Geometry check sheet. Reference: the model listing, model coordinates, mm. Face numbers are marked on the shaded views. A direction names the side the tool comes from. Give positions to 0.01 mm unless a question says otherwise; leave off trailing zeros. Order: outer loops, then holes, each group sorted by start corner. A loop starts at its lowest first (then second) coordinate and runs counter-clockwise, first axis right, second up. Notation, with made-up numbers: M 35,-1 L 68,-1 A23 cw 68,19 Z; hole C -29.75,38.25 d10. An arc over 180 degrees is marked long. Put each result on its own line as item: value. Start each with the question number.
Q1. Section check B-B on z = -8. Record the cut outline in (x, y), then the cut area to 3 significant figures.
Q2. Material ranges on L1, parallel to X at y = 87, z = -15.5; L2, parallel to X at y = 87, z = -22; L3, parallel to Y at x = 1, z = 1, recorded low to high.
Q3. Go/stop test with flat-tipped pins: pin 1 (6 mm diameter, centred on y = 72.5, z = 5.5, fed in from -X); pin 2 (12 mm diameter, centred on x = 27.5, z = -18.5, fed in from +Y); pin 3 (1 mm diameter, centred on x = 40, y = 56.5, fed in from -Z). Record where each tip stops, or that it passes through.
Q4. Mould release check, pull along X, two halves, no side actions. Record for the marked faces 4, 5, 6 and 7: +X half, -X half, draft (parallel to the pull), parting line (faces both ways), or undercut.
Q5. Access from +Z, -Z, +X, -X, +Y, -Y to the whole of each face (thin tool, end or side, straight path). Record for the marked faces 1, 2 and 3.
Q6. Section check C-C on x = -34.5. Record the cut outline in (y, z), then the cut area to 3 significant figures.
Q7. Section check A-A on y = 38. Record the cut outline in (x, z).
Q8. Section check D-D on x = -14.5. Record the cut outline in (y, z).
```python
from build123d import *

# Parameters (mm, degrees)
EXTRUDE_2_DEPTH          = 90
CUT_EXTRUDE_1_DEPTH      = 114.317207464
CUT_EXTRUDE_1_DEPTH_BACK = 114.317207464
EXTRUDE_3_DEPTH          = 8
SKETCH_8_OUTSIDE_W       = 163.572
SKETCH_8_OUTSIDE_H       = 147.98
SKETCH_8_OUTSIDE_W_2     = 117.820012314
SKETCH_8_OUTSIDE_H_2     = 106.962978805
CUT_EXTRUDE_2_DEPTH      = 117.531399887
SKETCH_9_R               = 2
CUT_EXTRUDE_3_DEPTH      = 115.369004136
SKETCH_10_W              = 117.820012314
SKETCH_10_H              = 8
CUT_EXTRUDE_4_DEPTH      = 20
CUT_EXTRUDE_6_DEPTH      = 5
CHAMFER_1_SIZE           = 8


with BuildPart() as part:
    # 草图5 → 拉伸-薄壁2 (new body)
    with BuildSketch(Plane(origin=(0, 0, 0), x_dir=(1, 0, 0), z_dir=(0, 1, 0))):
        Polygon((-58.910006157, 27.470187013), (0, 0), (58.910006157, 27.470187013), (63.136188775, 18.407109143), (0, -11.03377919), (-63.136188775, 18.407109143), align=None)
    extrude(amount=EXTRUDE_2_DEPTH)

    # 草图6 → 切除-拉伸1 (cut, two sides: drawn at the far end of the back side and taken through both)
    with BuildSketch(Plane(origin=(0, 0, 0), x_dir=(0, 0, -1), z_dir=(1, 0, 0)).offset(-CUT_EXTRUDE_1_DEPTH_BACK)):
        Polygon((-11.03377919, 0), (27.470187013, 26.960767386), (27.470187013, 0), align=None)
        Polygon((27.470187013, 90), (-11.03377919, 63.039232614), (-11.03377919, 90), align=None)
    extrude(amount=CUT_EXTRUDE_1_DEPTH + CUT_EXTRUDE_1_DEPTH_BACK, mode=Mode.SUBTRACT)

    # 草图7 → 凸台-拉伸3 (add)
    with BuildSketch(Plane(origin=(0, 47.484140436, 33.248753079), x_dir=(1, 0, 0), z_dir=(0, 0.8191520442889949, 0.5735764363510419))):
        Polygon((63.136188775, 63.06016396), (58.910006157, 74.12413912), (58.910006157, 94.12413912), (-58.910006157, 94.12413912), (-58.910006157, 74.12413912), (-63.136188775, 63.06016396), (0, 27.119475614), align=None)
    extrude(amount=EXTRUDE_3_DEPTH)

    # 草图8 outside → 切除-拉伸2 (cut, through all)
    with BuildSketch(Plane(origin=(0, 54.03735679, 37.837364569), x_dir=(1, 0, 0), z_dir=(0, 0.8191520442889948, 0.5735764363510418))):
        with Locations((0, 42.543)):
            Rectangle(SKETCH_8_OUTSIDE_W, SKETCH_8_OUTSIDE_H)
        with Locations((0, 40.642649718)):
            Rectangle(SKETCH_8_OUTSIDE_W_2, SKETCH_8_OUTSIDE_H_2, mode=Mode.SUBTRACT)
    extrude(amount=-CUT_EXTRUDE_2_DEPTH, mode=Mode.SUBTRACT)

    # 草图9 → 切除-拉伸3 (cut, through all)
    with BuildSketch(Plane(origin=(0, 47.484140436, 33.248753079), x_dir=(1, 0, 0), z_dir=(0, -0.8191520442889949, -0.5735764363510419))):
        with Locations(Location((-45, -74.12413912, 0), (0, 0, 270))):
            Circle(SKETCH_9_R)
        with Locations(Location((45, -74.12413912, 0), (0, 0, 270))):
            Circle(SKETCH_9_R)
    extrude(amount=-CUT_EXTRUDE_3_DEPTH, mode=Mode.SUBTRACT)

    # 草图10 → 切除-拉伸4 (cut)
    with BuildSketch(Plane(origin=(0, 47.484140436, 33.248753079), x_dir=(1, 0, 0), z_dir=(0, -0.8191520442889949, -0.5735764363510419))):
        with Locations((0, -90.12413912)):
            Rectangle(SKETCH_10_W, SKETCH_10_H)
    extrude(amount=-CUT_EXTRUDE_4_DEPTH, mode=Mode.SUBTRACT)

    # 草图11 → 切除-拉伸6 (cut)
    with BuildSketch(Plane(origin=(0, 47.484140436, 33.248753079), x_dir=(1, 0, 0), z_dir=(0, -0.8191520442889949, -0.5735764363510419))):
        Polygon((-58.910006157, -86.12413912), (58.910006157, -86.12413912), (58.910006157, -74.12413912), (0, -40.589232866), (-58.910006157, -74.12413912), align=None)
    extrude(amount=-CUT_EXTRUDE_6_DEPTH, mode=Mode.SUBTRACT)

    # 倒角1
    chamfer_1_edges = [part.edges().sort_by_distance(p)[0] for p in [
        (-58.910006157, 102.207405524, -33.571764708),
        (58.910006157, 102.207405524, -33.571764708),
    ]]
    chamfer(chamfer_1_edges, length=CHAMFER_1_SIZE)


solid = part.part
```
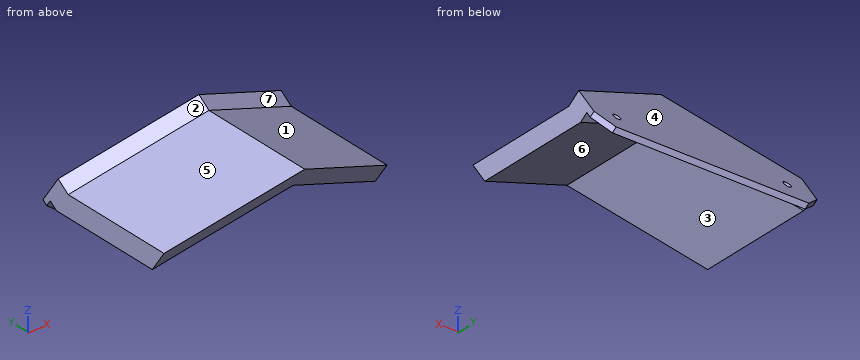
Results found:
1. outline: M -50.66,86.13 L -40.82,76.37 L -40.82,13.33 L -17.16,13.33 L -17.16,76.37 L -23.31,82.47 L 23.31,82.47 L 17.16,76.37 L 17.16,13.33 L 40.82,13.33 L 40.82,76.37 L 50.66,86.13 Z
1. area: 3,630 mm^2
2. L1: x = -58.91 to -38.66, 38.66 to 58.91
2. L2: x = -58.91 to -48.02, 48.02 to 58.91
2. L3: y = 7.03 to 73.19, 76.17 to 79.83
3. pin 1: stops at x = -22.77
3. pin 2: stops at y = 97.69
3. pin 3: stops at z = -18.89
4. face 4: draft
4. face 5: -X half
4. face 6: undercut
4. face 7: +X half
5. face 1: +Z, +X, -Y
5. face 2: +Z, -X, -Y
5. face 3: -Z, -Y
6. outline: M 11.26,-5.05 L 18.99,-16.09 L 82.03,-16.09 L 86.13,-13.22 L 100.98,-34.43 L 103.44,-32.71 L 80.86,-0.47 L 74.3,-5.05 Z
6. area: 881 mm^2
7. outline: M -58.91,-27.47 L 0,0 L 58.91,-27.47 L 58.91,-16.44 L 0,11.03 L -58.91,-16.44 Z
8. outline: M 4.73,4.27 L 12.46,-6.76 L 75.5,-6.76 L 79.6,-3.89 L 100.98,-34.43 L 103.44,-32.71 L 74.33,8.86 L 67.77,4.27 Z
